Part model, mm, in its own coordinate system. Face numbers are marked on the shaded views. Round coordinates to 2 decimals unless told otherwise and drop trailing zeros. Loops run counter-clockwise (first coordinate to the right, second up) from the corner with the lowest first, then second, coordinate; pieces in that order, holes last.
(1) Flat gauge pins, fed straight in: pin 1 (12 mm diameter, centred on y = 328.5, z = 2.5, fed in from -X); pin 2 (1.5 mm diameter, centred on x = 5.5, z = -18, fed in from -Y); pin 3 (5 mm diameter, centred on x = -93.5, z = -12, fed in from +Y). Where does each tip first touch, or does it go through?
(2) Cut at A-A on x = 0. List the corners of the cut face in (y, z), then the cut area to 3 significant figures.
(3) Probe probe 1 along Y at (x, z) = (3, 27); probe 2 along Y at (x, z) = (13, -13); probe 3 along Y at (x, z) = (30.5, -14). List the from-to ranges inside material, lowest first.
(4) Cut at C-C on y = 79.5. List the corners of the cut face in (x, z).
(5) Cut at D-D on x = -78. List the corners of the cut face in (y, z), then the cut area to 3 significant figures.
(6) Mould opens along X. For the marked faces 1, 2, 3 and 4 say: +X half, -X half, draft (parallel to the pull), parting line (faces both ways), or undercut.
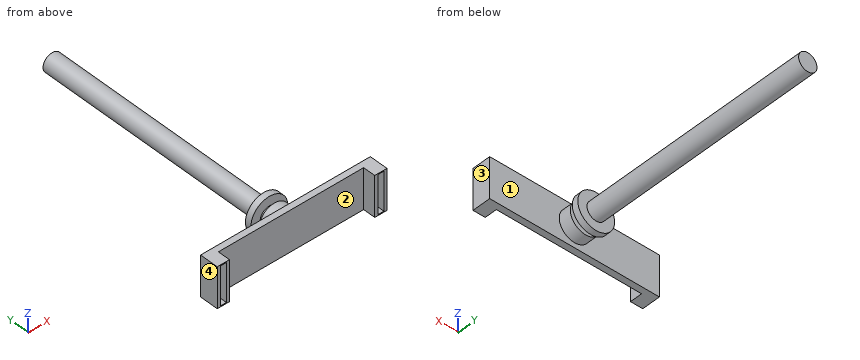
from build123d import *

# Parameters (mm, degrees)
BOSS_EXTRUDE1_DEPTH      = 33
BOSS_EXTRUDE1_DEPTH_BACK = 33
SKETCH2_W                = 10
SKETCH2_H                = 63
CUT_EXTRUDE1_DEPTH       = 20
SKETCH3_R                = 25
BOSS_EXTRUDE2_DEPTH      = 20
SKETCH4_R                = 15
BOSS_EXTRUDE3_DEPTH      = 400
SKETCH5_R                = 30
BOSS_EXTRUDE4_DEPTH      = 10


with BuildPart() as part:
    # Sketch1 → Boss-Extrude1 (new, two sides: drawn at the far end of the back side and taken through both)
    with BuildSketch(Plane.XY.offset(-BOSS_EXTRUDE1_DEPTH_BACK)):
        Polygon((-138.5, 0), (138.5, 0), (138.5, -30), (118.5, -30), (118.5, -10), (-118.5, -10), (-118.5, -30), (-138.5, -30), align=None)
    extrude(amount=BOSS_EXTRUDE1_DEPTH + BOSS_EXTRUDE1_DEPTH_BACK)

    # Sketch2 → Cut-Extrude1 (cut)
    with BuildSketch(Plane.XZ.offset(30)):
        with Locations((-128.5, 0)):
            Rectangle(SKETCH2_W, SKETCH2_H)
        with Locations((128.5, 0)):
            Rectangle(SKETCH2_W, SKETCH2_H)
    extrude(amount=-CUT_EXTRUDE1_DEPTH, mode=Mode.SUBTRACT)

    # Sketch3 → Boss-Extrude2 (add)
    with BuildSketch(Plane(origin=(0, 0, 0), x_dir=(1, 0, 0), z_dir=(0, 1, 0))):
        with Locations(Location((0, 0, 0), (0, 0, 180))):
            Circle(SKETCH3_R)
    extrude(amount=BOSS_EXTRUDE2_DEPTH)

    # Sketch4 → Boss-Extrude3 (add)
    with BuildSketch(Plane(origin=(0, 20, 0), x_dir=(1, 0, 0), z_dir=(0, 1, 0))):
        with Locations(Location((0, 0, 0), (0, 0, 180))):
            Circle(SKETCH4_R)
    extrude(amount=BOSS_EXTRUDE3_DEPTH)

    # Sketch5 → Boss-Extrude4 (add)
    with BuildSketch(Plane(origin=(0, 29, 0), x_dir=(1, 0, 0), z_dir=(0, 1, 0))):
        with Locations(Location((0, 0, 0), (0, 0, 180))):
            Circle(SKETCH5_R)
    extrude(amount=BOSS_EXTRUDE4_DEPTH)


solid = part.part
Final values:
1. pin 1: stops at x = -15
1. pin 2: stops at y = -10
1. pin 3: stops at y = 0
2. outline: (-10, -33) - (0, -33) - (0, -25) - (20, -25) - (20, -15) - (29, -15) - (29, -30) - (39, -30) - (39, -15) - (420, -15) - (420, 15) - (39, 15) - (39, 30) - (29, 30) - (29, 15) - (20, 15) - (20, 25) - (0, 25) - (0, 33) - (-10, 33) - close
2. area: 14,000 mm2
3. probe 1: y = -10 to 0, 29 to 39
3. probe 2: y = -10 to 20, 29 to 39
3. probe 3: y = -10 to 0
4. outline: circle Ø30 at (0, 0)
5. outline: (-10, -33) - (0, -33) - (0, 33) - (-10, 33) - close
5. area: 660 mm2
6. face 1: draft
6. face 2: undercut
6. face 3: +X half
6. face 4: -X half
